from build123d import *

# Parameters (mm, degrees)
BOSS_EXTRUDE1_DEPTH = 5.08
FILLET1_R           = 8.89
SKETCH2_R           = 3.96875
CUT_EXTRUDE1_DEPTH  = 6.08
SKETCH3_R           = 1.5875
CUT_EXTRUDE2_DEPTH  = 6.08
BOSS_EXTRUDE3_DEPTH = 1.905


with BuildPart() as part:
    # Sketch1 → Boss-Extrude1 (new body)
    with BuildSketch(Plane.XY):
        Polygon((0, 184.15), (60.96, 123.19), (60.96, 80.01), (0, 19.05), (19.05, 0), (80.01, 60.96), (123.19, 60.96), (184.15, 0), (203.2, 19.05), (142.24, 80.01), (142.24, 123.19), (203.2, 184.15), (184.15, 203.2), (123.19, 142.24), (80.01, 142.24), (19.05, 203.2), align=None)
    extrude(amount=BOSS_EXTRUDE1_DEPTH)

    # Fillet1
    fillet1_edges = [part.edges().sort_by_distance(p)[0] for p in [
        (19.05, 203.2, 2.54),
        (80.01, 142.24, 2.54),
        (123.19, 142.24, 2.54),
        (184.15, 203.2, 2.54),
        (203.2, 184.15, 2.54),
        (142.24, 123.19, 2.54),
        (142.24, 80.01, 2.54),
        (203.2, 19.05, 2.54),
        (184.15, 0, 2.54),
        (123.19, 60.96, 2.54),
        (80.01, 60.96, 2.54),
        (19.05, 0, 2.54),
        (0, 19.05, 2.54),
        (60.96, 80.01, 2.54),
        (60.96, 123.19, 2.54),
        (0, 184.15, 2.54),
    ]]
    fillet(fillet1_edges, radius=FILLET1_R)

    # Sketch2 → Cut-Extrude1 (cut, through all)
    with BuildSketch(Plane.XY.offset(5.08)):
        with Locations((127.508, 86.36)):
            Circle(SKETCH2_R)
        with Locations((127.508, 116.84)):
            Circle(SKETCH2_R)
        with Locations((75.692, 86.36)):
            Circle(SKETCH2_R)
        with Locations((75.692, 116.84)):
            Circle(SKETCH2_R)
    extrude(amount=-CUT_EXTRUDE1_DEPTH, mode=Mode.SUBTRACT)

    # Sketch3 → Cut-Extrude2 (cut, through all)
    with BuildSketch(Plane.XY.offset(5.08)):
        with Locations((184.688815367, 184.700672391)):
            Circle(SKETCH3_R)
        with Locations((18.511184633, 184.700672391)):
            Circle(SKETCH3_R)
        with Locations((18.511184633, 18.499327609)):
            Circle(SKETCH3_R)
        with Locations((184.688815367, 18.499327609)):
            Circle(SKETCH3_R)
    extrude(amount=-CUT_EXTRUDE2_DEPTH, mode=Mode.SUBTRACT)

    # Sketch5 → Boss-Extrude3 (add, symmetric)
    with BuildSketch(Plane(origin=(101.6, 0, 0), x_dir=(0, 0, -1), z_dir=(1, 0, 0))):
        with BuildLine():
            Line((-5.08, 99.695), (-5.08, 103.505))
            Line((-5.08, 103.505), (-9.652, 103.505))
            ThreePointArc((-9.652, 103.505), (-11.557, 101.6), (-9.652, 99.695))
            Line((-9.652, 99.695), (-5.08, 99.695))
        make_face()
    extrude(amount=BOSS_EXTRUDE3_DEPTH, both=True)


solid = part.part
Design review of the part built by this model. Coordinates are the model's own, in mm. A direction names the side the tool comes from. Give positions to 0.01 mm unless a question says otherwise; leave off trailing zeros. Write each loop counter-clockwise with the first axis right and the second up, starting at its lowest first coordinate (ties: lowest second). Pieces come first, ordered by that corner, then holes. Notation, with made-up numbers: M -32.75,88.25 L 12.25,88.25 A38 ccw 12.25,126.25 Z; hole C -17.5,-26.5 d1. An arc over 180 degrees is marked long. Return JSON: item names as keys, results as strings. Group by question number.
Item 1: Clearance check with flat-ended pins moving along their axes: pin 1 Ø2.5 at (y, z) = (98.5, 2) entering from +X; pin 2 Ø1.5 at (x, z) = (110.5, 1.5) entering from -Y; pin 3 Ø1 at (x, z) = (50, 7.5) entering from +Y; pin 4 Ø1.9 at (x, z) = (102.5, 7) entering from +Y (3 decimals). State where each tip first meets the part, or that it passes through.
Item 2: The part is to be moulded in two halves that separate along Y. For faces 4 (the cylindrical face through (80.245, 60.264, 2.576)), 5 (the cylindrical face through (80.336, 142.898, 2.576)), 6 (the flat face through (170.51, 151.46, 2.5)), 7 (the cylindrical face through (129.642, 120.186, 2.576)), say which applies: pulls with the +Y half, pulls with the -Y half, needs draft (parallel to the pull), parting line crosses it, or undercut.
Item 3: Tool access review of faces 1 (the cylindrical face through (60.302, 80.336, 2.576)), 2 (the flat face through (51.01, 31.96, 2.5)), 3 (the cylindrical face through (122.955, 142.936, 2.576)): name each direction out of +Z, -Z, +X, -X, +Y, -Y from which nothing blocks a thin tool from reaching the whole face with its end or side.
Item 4: Take a section at B-B (x = 154.5). Give the boundary of the cut face in (y, z), plus the area to 3 significant figures.
Item 5: Take a section at C-C (z = 7). Give the boundary of the cut face in (x, y) (3 decimals), plus the area to 3 significant figures.
Item 6: Wall thickness on line 1 along Y through (x, z) = (77.5, 1.75); line 2 along Z through (x, y) = (177, 19.5); line 3 along Y through (x, z) = (153, 1.75): over which ranges is each line inside the solid? List them lowest first.
Item 7: Take a section at A-A (y = 116.84). Give the boundary of the cut face in (x, z).
Return value:
{
 "1": {"pin 1": "stops at x = 142.24", "pin 2": "stops at y = 60.96", "pin 3": "passes through", "pin 4": "stops at y = 103.505"},
 "2": {"face 4": "pulls with the -Y half", "face 5": "pulls with the +Y half", "face 6": "undercut", "face 7": "undercut"},
 "3": {"face 1": "+Z, -Z, -X", "face 2": "+Z, -Z, -Y", "face 3": "+Z, -Z, +Y"},
 "4": {"outline": "M 29.65,0 L 67.75,0 L 67.75,5.08 L 29.65,5.08 Z; M 135.45,0 L 173.55,0 L 173.55,5.08 L 135.45,5.08 Z", "area": "387 mm2"},
 "5": {"outline": "M 99.695,99.695 L 103.505,99.695 L 103.505,103.505 L 99.695,103.505 Z", "area": "14.5 mm2"},
 "6": {"line 1": "y = 58.45 to 82.83, 89.89 to 113.31, 120.37 to 144.75", "line 2": "z = 0 to 5.08", "line 3": "y = 31.15 to 69.25, 133.95 to 172.05"},
 "7": {"outline": "M 60.96,0 L 71.72,0 L 71.72,5.08 L 60.96,5.08 Z; M 79.66,0 L 123.54,0 L 123.54,5.08 L 79.66,5.08 Z; M 131.48,0 L 142.24,0 L 142.24,5.08 L 131.48,5.08 Z"}
}
